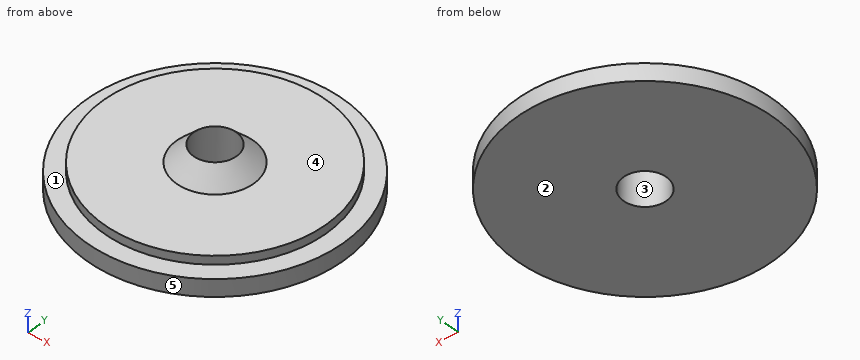
from build123d import *

# Parameters (mm, degrees)
F0_R     = 15
F0_R_2   = 2.5
F1_DEPTH = 2
F2_R     = 13
F2_R_2   = 2.5
F3_DEPTH = 1
F4_R     = 4.5
F4_R_2   = 2.5
F5_DEPTH = 2
F6_SIZE2 = 1.99999
F6_SIZE  = 1.99999


# Not quite as in the source:
# - a fillet or chamfer is up to 0.001 mm smaller than in the source, because OpenCascade refuses the exact size


with BuildPart() as f1:
    # F0 (on Top) → F1 (new body)
    with BuildSketch(Plane.XY):
        Circle(F0_R)
        Circle(F0_R_2, mode=Mode.SUBTRACT)
    extrude(amount=F1_DEPTH)

    # F2 (on face) → F3 (join)
    with BuildSketch(Plane.XY.offset(2)):
        Circle(F2_R)
        Circle(F2_R_2, mode=Mode.SUBTRACT)
    extrude(amount=F3_DEPTH)

    # F4 (on face) → F5 (join)
    with BuildSketch(Plane.XY.offset(3)):
        Circle(F4_R)
        Circle(F4_R_2, mode=Mode.SUBTRACT)
    extrude(amount=F5_DEPTH)

    # F6 (size 2 and 2 in the source; OpenCascade refuses exactly that, so slightly less here)
    f6_edges = [f1.edges().sort_by_distance(p)[0] for p in [
        (-4.5, 0, 5),
    ]]
    chamfer(f6_edges, length=F6_SIZE, length2=F6_SIZE2)


solid = f1.part
Check sheet for the modelled part. Datum: model origin and axes. Units: mm. Face numbers are marked on the shaded views. A direction names the side the tool comes from. Give positions to 0.01 mm unless a question says otherwise; leave off trailing zeros. Write each loop counter-clockwise with the first axis right and the second up, starting at its lowest first coordinate (ties: lowest second). Pieces come first, ordered by that corner, then holes. Notation, with made-up numbers: M 41,44.25 L 97,44.25 A23 cw 97,65.25 Z; hole C 42.25,-23 d2. An arc over 180 degrees is marked long. Use one line per item in the form item = value.
(1) Draft check along Y on the marked faces 3, 4 and 5. Enter one of: pulls with the +Y half, pulls with the -Y half, needs draft (parallel to the pull), parting line crosses it, or undercut.
Answer block:
face_3 = undercut
face_4 = needs draft
face_5 = parting line crosses it
(2) Section check C-C on z = 1.35. Record the boundary of the cut face in (x, y), plus the area to 3 significant figures.
Answer block:
outline = C 0,0 d30; hole C 0,0 d5
area = 687 mm2
(3) Material ranges on line 1 along Z through (x, y) = (-6, 0.75); line 2 along Z through (x, y) = (-3, 13.5); line 3 along Y through (x, z) = (0, 3.4), recorded low to high.
Answer block:
line_1 = 0 to 3
line_2 = 0 to 2
line_3 = -4.1 to -2.5, 2.5 to 4.1
(4) Section check D-D on y = 11.75. Record the boundary of the cut face in (x, z), plus the area to 3 significant figures.
Answer block:
outline = M -9.32,0 L 9.32,0 L 9.32,2 L 5.56,2 L 5.56,3 L -5.56,3 L -5.56,2 L -9.32,2 Z
area = 48.4 mm2
(5) Tool access check on the marked faces 1 and 2. Record the directions out of +Z, -Z, +X, -X, +Y, -Y that give a thin tool (end or side, any length) a straight path to the whole face; none if there is none.
Answer block:
face_1 = +Z
face_2 = -Z, +X, -X, +Y, -Y
